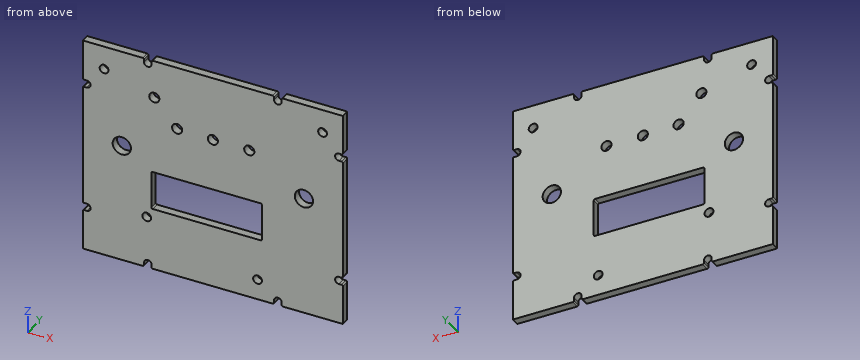
from build123d import *

# Parameters (mm, degrees)
SKETCH1_W                       = 101.6
SKETCH1_H                       = 85.725
BOSS_EXTRUDE1_DEPTH             = 3.175
F_29_0_136_DIAMETER_HOLE1_D     = 3.4544
F_9_32_0_28125_DIAMETER_HOLE1_D = 7.14375
F_5_32_0_15625_DIAMETER_HOLE1_D = 3.96875
SKETCH8_W                       = 43.18
SKETCH8_H                       = 15.24
CUT_EXTRUDE1_DEPTH              = 67.542576831
CUT_EXTRUDE2_DEPTH              = 67.542576831
FILLET1_R                       = 0.508
CUT_EXTRUDE3_DEPTH              = 67.542576831
FILLET2_R                       = 0.508


with BuildPart() as part:
    # Sketch1 → Boss-Extrude1 (new body)
    with BuildSketch(Plane(origin=(0, 0, 0), x_dir=(1, 0, 0), z_dir=(0, 1, 0))):
        Rectangle(SKETCH1_W, SKETCH1_H)
    extrude(amount=BOSS_EXTRUDE1_DEPTH)

    # #29 (0.136) Diameter Hole1 (through all)
    with Locations(Plane(origin=(0, 3.175, 0), x_dir=(1, 0, 0), z_dir=(0, 1, 0))):
        with Locations((-25.8318, 22.2123), (17.4498, 34.7853), (42.8498, -33.6423), (-42.4688, -33.6423)):
            Hole(F_29_0_136_DIAMETER_HOLE1_D / 2)

    # 9/32 (0.28125) Diameter Hole1 (through all)
    with Locations(Plane(origin=(0, 3.175, 0), x_dir=(1, 0, 0), z_dir=(0, 1, 0))):
        with Locations((-35.56, -4.1275), (35.56, -4.1275)):
            Hole(F_9_32_0_28125_DIAMETER_HOLE1_D / 2)

    # 5/32 (0.15625) Diameter Hole1 (through all)
    with Locations(Plane(origin=(0, 3.175, 0), x_dir=(1, 0, 0), z_dir=(0, 1, 0))):
        with Locations((-22.86, -27.8765), (-13.942192497, -17.744307503), (0, -17.4625), (14.224, -17.4625)):
            Hole(F_5_32_0_15625_DIAMETER_HOLE1_D / 2)

    # Sketch8 → Cut-Extrude1 (cut, through all)
    with BuildSketch(Plane(origin=(0, 3.175, 0), x_dir=(1, 0, 0), z_dir=(0, 1, 0))):
        with Locations((-2.413, 10.6045)):
            Rectangle(SKETCH8_W, SKETCH8_H)
    extrude(amount=-CUT_EXTRUDE1_DEPTH, mode=Mode.SUBTRACT)

    # Sketch9 → Cut-Extrude2 (cut, through all)
    with BuildSketch(Plane(origin=(0, 3.175, 0), x_dir=(1, 0, 0), z_dir=(0, 1, 0))):
        with BuildLine():
            Line((-49.2125, 26.8732), (-50.8, 26.8732))
            Line((-50.8, 26.8732), (-50.8, 23.9268))
            Line((-50.8, 23.9268), (-49.2125, 23.9268))
            ThreePointArc((-49.2125, 23.9268), (-47.7393, 25.4), (-49.2125, 26.8732))
        make_face()
        with BuildLine():
            Line((-49.2125, -23.9268), (-50.8, -23.9268))
            Line((-50.8, -23.9268), (-50.8, -26.8732))
            Line((-50.8, -26.8732), (-49.2125, -26.8732))
            ThreePointArc((-49.2125, -26.8732), (-47.7393, -25.4), (-49.2125, -23.9268))
        make_face()
        with BuildLine():
            Line((49.2125, -26.8732), (50.8, -26.8732))
            Line((50.8, -26.8732), (50.8, -23.9268))
            Line((50.8, -23.9268), (49.2125, -23.9268))
            ThreePointArc((49.2125, -23.9268), (47.7393, -25.4), (49.2125, -26.8732))
        make_face()
        with BuildLine():
            Line((50.8, 26.8732), (50.8, 23.9268))
            Line((50.8, 23.9268), (49.2125, 23.9268))
            ThreePointArc((49.2125, 23.9268), (47.7393, 25.4), (49.2125, 26.8732))
            Line((49.2125, 26.8732), (50.8, 26.8732))
        make_face()
    extrude(amount=-CUT_EXTRUDE2_DEPTH, mode=Mode.SUBTRACT)

    # Fillet1
    fillet1_edges = [part.edges().sort_by_distance(p)[0] for p in [
        (-50.8, 1.5875, -26.8732),
        (-50.8, 1.5875, 26.8732),
        (-50.8, 1.5875, 23.9268),
        (50.8, 1.5875, 23.9268),
        (50.8, 1.5875, 26.8732),
        (50.8, 1.5875, -26.8732),
        (50.8, 1.5875, -23.9268),
        (-24.003, 1.5875, -2.9845),
        (-24.003, 1.5875, -18.2245),
        (19.177, 1.5875, -18.2245),
        (19.177, 1.5875, -2.9845),
        (-50.8, 1.5875, -23.9268),
    ]]
    fillet(fillet1_edges, radius=FILLET1_R)

    # Sketch10 → Cut-Extrude3 (cut, through all)
    with BuildSketch(Plane(origin=(0, 3.175, 0), x_dir=(1, 0, 0), z_dir=(0, 1, 0))):
        with BuildLine():
            Line((-23.9268, 41.275), (-23.9268, 42.8625))
            Line((-23.9268, 42.8625), (-26.8732, 42.8625))
            Line((-26.8732, 42.8625), (-26.8732, 41.275))
            ThreePointArc((-26.8732, 41.275), (-25.4, 39.8018), (-23.9268, 41.275))
        make_face()
        with BuildLine():
            Line((26.8732, -41.275), (26.8732, -42.8625))
            Line((26.8732, -42.8625), (23.9268, -42.8625))
            Line((23.9268, -42.8625), (23.9268, -41.275))
            ThreePointArc((23.9268, -41.275), (25.4, -39.8018), (26.8732, -41.275))
        make_face()
        with BuildLine():
            Line((-23.9268, -41.275), (-23.9268, -42.8625))
            Line((-23.9268, -42.8625), (-26.8732, -42.8625))
            Line((-26.8732, -42.8625), (-26.8732, -41.275))
            ThreePointArc((-26.8732, -41.275), (-25.4, -39.8018), (-23.9268, -41.275))
        make_face()
        with BuildLine():
            Line((26.8732, 42.8625), (23.9268, 42.8625))
            Line((23.9268, 42.8625), (23.9268, 41.275))
            ThreePointArc((23.9268, 41.275), (25.4, 39.8018), (26.8732, 41.275))
            Line((26.8732, 41.275), (26.8732, 42.8625))
        make_face()
    extrude(amount=-CUT_EXTRUDE3_DEPTH, mode=Mode.SUBTRACT)

    # Fillet2
    fillet2_edges = [part.edges().sort_by_distance(p)[0] for p in [
        (-26.8732, 1.5875, -42.8625),
        (-23.9268, 1.5875, -42.8625),
        (26.8732, 1.5875, -42.8625),
        (23.9268, 1.5875, -42.8625),
        (-23.9268, 1.5875, 42.8625),
        (-26.8732, 1.5875, 42.8625),
        (26.8732, 1.5875, 42.8625),
        (23.9268, 1.5875, 42.8625),
    ]]
    fillet(fillet2_edges, radius=FILLET2_R)


solid = part.part
Build history of the part. All positions in model axes, mm. Coordinates: 2 decimals unless noted, no trailing zeros. Write each loop counter-clockwise with the first axis right and the second up, starting at its lowest first coordinate (ties: lowest second). Pieces come first, ordered by that corner, then holes.
(1) Drill centre lines: line 1 (Z direction, x = -23, y = 0.9); line 2 (X direction, y = 3, z = 1); line 3 (X direction, y = 1.9, z = -8). Where is each one in solid material? Low to high.
(2) Cut at C-C on x = 35.56. List the corners of the cut face in (y, z) (1 decimal).
(3) Cut at B-B on z = -6. List the corners of the cut face in (x, y) (3 decimals).
(4) Cut at D-D on x = 25.4. List the corners of the cut face in (y, z) (3 decimals).
(5) Cut at A-A on x = 0. List the corners of the cut face in (y, z) (1 decimal), and give its area (3 significant figures).
Working result:
1. line 1: z = -42.86 to -18.22, -2.98 to 25.9, 29.86 to 42.86
1. line 2: x = -50.8 to -37.29, -33.83 to 33.83, 37.29 to 50.8
1. line 3: x = -50.8 to -24, 19.18 to 50.8
2. outline: (0, -42.9) - (3.2, -42.9) - (3.2, 0.6) - (0, 0.6) - close; (0, 7.7) - (3.2, 7.7) - (3.2, 42.9) - (0, 42.9) - close
3. outline: (-50.8, 0) - (-24.003, 0) - (-24.003, 3.175) - (-50.8, 3.175) - close; (19.177, 0) - (50.8, 0) - (50.8, 3.175) - (19.177, 3.175) - close
4. outline: (0, -39.802) - (3.175, -39.802) - (3.175, 39.802) - (0, 39.802) - close
5. outline: (0, -42.9) - (3.2, -42.9) - (3.2, -18.2) - (0, -18.2) - close; (0, -3) - (3.2, -3) - (3.2, 15.5) - (0, 15.5) - close; (0, 19.4) - (3.2, 19.4) - (3.2, 42.9) - (0, 42.9) - close
5. area: 211 mm2
